Print and shaded views of the part. All mm, measured from the part's lowest x, y and z. A direction names the side the tool comes from. Give positions to 0.01 mm unless a question says otherwise; leave off trailing zeros. Loops run counter-clockwise (first coordinate to the right, second up) from the corner with the lowest first, then second, coordinate; pieces in that order, holes last. Notation, with made-up numbers: M 1.5,84 L 41.5,84 A4 ccw 41.5,89 Z; hole C 38,15.5 d10. An arc over 180 degrees is marked long. Answer in a Markdown table with one row per item.
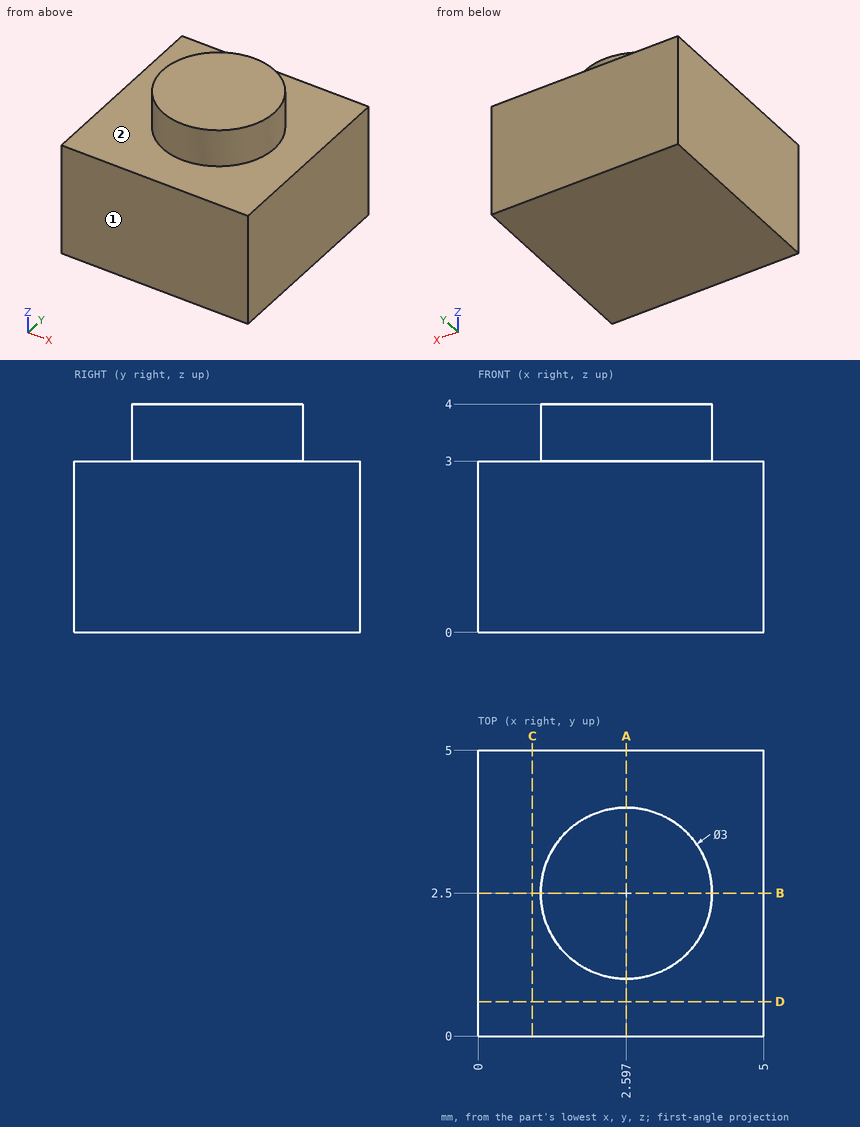
(1) Wall check: L1, parallel to Z at x = 4.3, y = 1.35; L2, parallel to Y at x = 3.35, z = 3.05. Give the ranges that are in metal, low to high.
Established:
| item | result |
|---|---|
| L1 | z = 0 to 3 |
| L2 | y = 1.2 to 3.8 |
(2) Saw through at B-B, the plane y = 2.5. Give the cut face in (x, z), and give its area (3 significant figures).
Established:
| item | result |
|---|---|
| outline | M 0,0 L 5,0 L 5,3 L 4.1,3 L 4.1,4 L 1.1,4 L 1.1,3 L 0,3 Z |
| area | 18.0 mm2 |
(3) Saw through at C-C, the plane x = 0.95. Give the cut face in (y, z), and give its area (3 significant figures).
Established:
| item | result |
|---|---|
| outline | M 0,0 L 5,0 L 5,3 L 0,3 Z |
| area | 15.0 mm2 |
(4) Which spindle directions (+Z, -Z, +X, -X, +Y, -Y) get a long thin tool onto all of the face, cutting with end or side? Do the marked faces 1 and 2. Say none if no direction does.
Established:
| item | result |
|---|---|
| face 1 | +Z, -Z, +X, -X, -Y |
| face 2 | +Z |
(5) Saw through at A-A, the plane x = 2.6. Give the cut face in (y, z).
Established:
| item | result |
|---|---|
| outline | M 0,0 L 5,0 L 5,3 L 4,3 L 4,4 L 1,4 L 1,3 L 0,3 Z |
